```python
from build123d import *

# Parameters (mm, degrees)
BOSS_EXTRUDE1_DEPTH = 7.62


with BuildPart() as part:
    # Sketch3 → Boss-Extrude1 (new body)
    with BuildSketch(Plane.XY):
        with BuildLine():
            Line((-8.798818102, 5.08), (-91.348818102, 5.08))
            ThreePointArc((-91.348818102, 5.08), (-98.268424141, 9.984696391), (-106.497636205, 7.931147458))
            Line((-106.497636205, 7.931147458), (-106.497636205, 6.35))
            Line((-106.497636205, 6.35), (-100.003810414, 6.35))
            Line((-100.003810414, 6.35), (-96.337636205, 0))
            Line((-96.337636205, 0), (-100.003810414, -6.35))
            Line((-100.003810414, -6.35), (-106.497636205, -6.35))
            Line((-106.497636205, -6.35), (-106.497636205, -7.931147458))
            ThreePointArc((-106.497636205, -7.931147458), (-98.268424141, -9.984696391), (-91.348818102, -5.08))
            Line((-91.348818102, -5.08), (-8.798818102, -5.08))
            ThreePointArc((-8.798818102, -5.08), (10.16, 0), (-8.798818102, 5.08))
        make_face()
        Polygon((7.332348419, 0), (3.666174209, 6.35), (-3.666174209, 6.35), (-7.332348419, 0), (-3.666174209, -6.35), (3.666174209, -6.35), align=None, mode=Mode.SUBTRACT)
    extrude(amount=BOSS_EXTRUDE1_DEPTH)


solid = part.part
```
Geometry: final body of the model. Coordinates: model frame, mm. A direction names the side the tool comes from. Give positions to 0.01 mm unless a question says otherwise; leave off trailing zeros. Write each loop counter-clockwise with the first axis right and the second up, starting at its lowest first coordinate (ties: lowest second). Pieces come first, ordered by that corner, then holes.
1. Section query D-D, the plane x = -24.5. Return loops of the section in (y, z), then the cut area to 3 significant figures.
2. Draft query along X for faces 4 (the flat face through (-49, 0, 0)), 5 (the flat face through (0, 6.35, 4)), 6 (the flat face through (5.474, -3.219, 3.757)), 7 (the flat face through (-98.196, 3.219, 3.757)). Return one class per face: released by +X, released by -X, zero draft, split by the parting line, or undercut.
3. Line query: probe 1 along X at (y, z) = (0, 3); probe 2 along Y at (x, z) = (-100, 7.25); probe 3 along X at (y, z) = (-5.5, 5.75). Output: solid intervals per line, ascending.
4. Pin query (flat end, axial travel): P1, Ø4, axis at x = -39.5, z = 5.5, coming from the +Y side. Return the tip coordinate at first contact, or that it passes through.
5. Section query C-C, the plane y = 1. Return loops of the section in (x, z) (3 decimals), then the cut area to 3 significant figures.
6. Section query A-A, the plane z = 5.5. Return loops of the section in (x, y).
7. Reachability of faces 1 (the flat face through (-103, 6.35, 4)), 2 (the flat face through (-51, -5.08, 4)), 3 (the flat face through (-49, 5.08, 4)) from +Z, -Z, +X, -X, +Y, -Y: full face, straight path, thin tool, end or side. Return the list, or none.
8. Section query B-B, the plane x = 0. Return loops of the section in (y, z), then the cut area to 3 significant figures.
Computed:
1. outline: (-5.08, 0) - (5.08, 0) - (5.08, 7.62) - (-5.08, 7.62) - close
1. area: 77.4 mm2
2. face 4: zero draft
2. face 5: undercut
2. face 6: undercut
2. face 7: released by -X
3. probe 1: x = -96.34 to -7.33, 7.33 to 10.16
3. probe 2: y = -10.16 to -6.34, 6.34 to 10.16
3. probe 3: x = -99.51 to -91.61, -8.54 to -4.16, 4.16 to 8.54
4. P1: stops at y = 5.08
5. outline: (-96.915, 0) - (-6.755, 0) - (-6.755, 7.62) - (-96.915, 7.62) - close; (6.755, 0) - (10.111, 0) - (10.111, 7.62) - (6.755, 7.62) - close
5. area: 713 mm2
6. outline: (-106.5, -7.93) arc R10.16 ccw to (-91.35, -5.08) - (-8.8, -5.08) arc R10.16 ccw (long way) to (-8.8, 5.08) - (-91.35, 5.08) arc R10.16 ccw to (-106.5, 7.93) - (-106.5, 6.35) - (-100, 6.35) - (-96.34, 0) - (-100, -6.35) - (-106.5, -6.35) - close; hole (-7.33, 0) - (-3.67, -6.35) - (3.67, -6.35) - (7.33, 0) - (3.67, 6.35) - (-3.67, 6.35) - close
7. face 1: +Z, -Z, -X
7. face 2: +Z, -Z, -Y
7. face 3: +Z, -Z, +Y
8. outline: (-10.16, 0) - (-6.35, 0) - (-6.35, 7.62) - (-10.16, 7.62) - close; (6.35, 0) - (10.16, 0) - (10.16, 7.62) - (6.35, 7.62) - close
8. area: 58.1 mm2
